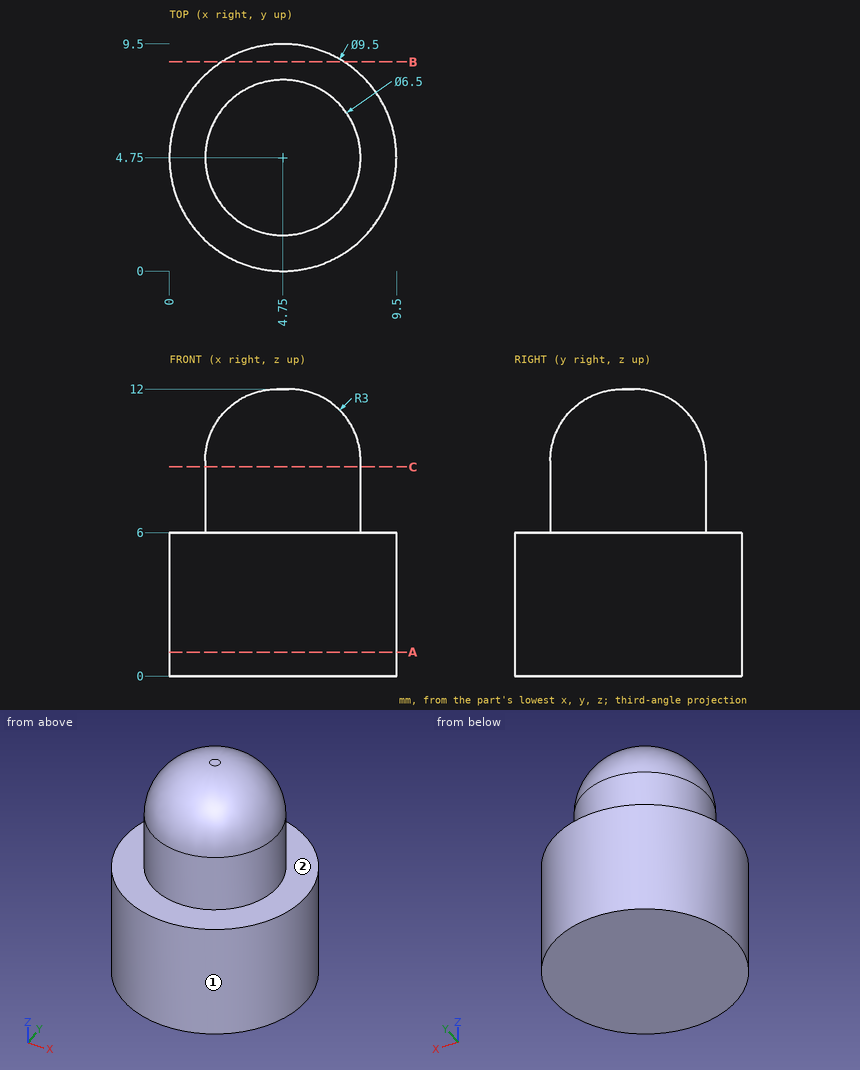
Could you check a few things on this drawing? It's one solid part, dimensions in mm from its lowest x, y, z. A direction names the side the tool comes from. Round coordinates to 2 decimals unless told otherwise and drop trailing zeros. Order: outer loops, then holes, each group sorted by start corner. A loop starts at its lowest first (then second) coordinate and runs counter-clockwise, first axis right, second up. Notation, with made-up numbers: M 12.25,44 L 35.25,44 A5 cw 35.25,48 Z; hole C 18.5,6 d3. An arc over 180 degrees is marked long. One line per item, written item: value.
(1) Which directions (+Z, -Z, +X, -X, +Y, -Y) give clear straight access to the entire face, cutting with the end or side of a thin tool? Please do the marked faces 1 and 2.
Ans:
face 1: +Z, -Z
face 2: +Z
(2) I need wall thicknesses on line 1 along Z through (x, y) = (8.5, 3); line 2 along X through (y, z) = (7.25, 10.5); line 3 along Z through (x, y) = (6, 6.75). Which ranges of each line are inside material? Lowest first, please. Write a range as from..to.
Ans:
line 1: z = 0..6
line 2: x = 3.39..6.11
line 3: z = 0..11.13
(3) Imagine slicing it at C-C (z = 8.75). Write out the boundary of the cut face in (x, y).
Ans:
outline: C 4.75,4.75 d6.5
(4) I'm going to push flat-ended pins straight in: P1, Ø3, axis at x = 3, y = 2, coming from the -Z side; P2, Ø4, axis at x = 7.5, y = 6, coming from the +Z side; P3, Ø4, axis at y = 7, z = 2.5, coming from the +X side. Where does each tip first touch, or does it pass through?
Ans:
P1: stops at z = 0
P2: stops at z = 11.9
P3: stops at x = 9.49
(5) Imagine slicing it at A-A (z = 1). Write out the boundary of the cut face in (x, y), and give its area (3 significant figures).
Ans:
outline: C 4.75,4.75 d9.5
area: 70.9 mm^2
(6) Imagine slicing it at B-B (y = 8.75). Write out the boundary of the cut face in (x, z), and give its area (3 significant figures).
Ans:
outline: M 2.19,0 L 7.31,0 L 7.31,6 L 2.19,6 Z
area: 30.7 mm^2
